Can you work these out from the model? Positions are in its coordinate system, mm. Face numbers are marked on the shaded views. Give positions to 0.01 mm unless a question says otherwise; leave off trailing zeros. Write each loop counter-clockwise with the first axis right and the second up, starting at its lowest first coordinate (ties: lowest second). Pieces come first, ordered by that corner, then holes. Notation, with made-up numbers: (55.25, 33.5) -> (86.25, 33.5) arc R24 cw to (86.25, 53.5) -> close; hole circle Ø9 at (12.5, 21.5). An arc over 180 degrees is marked (long way). One line per item, written item: value.
from build123d import *

# Parameters (mm, degrees)
F0_R     = 63.5
F1_DEPTH = 127


with BuildPart() as f1:
    # F0 (on Right) → F1 (new body)
    with BuildSketch(Plane.YZ):
        with BuildLine():
            Line((423.9281, 127), (-1100.0719, 127))
            ThreePointArc((-1100.0719, 127), (-1227.0719, 0), (-1100.0719, -127))
            Line((-1100.0719, -127), (423.9281, -127))
            ThreePointArc((423.9281, -127), (550.9281, 0), (423.9281, 127))
        make_face()
        with Locations((-1100.0719, 0)):
            Circle(F0_R, mode=Mode.SUBTRACT)
        with Locations((423.9281, 0)):
            Circle(F0_R, mode=Mode.SUBTRACT)
    extrude(amount=F1_DEPTH)


solid = f1.part
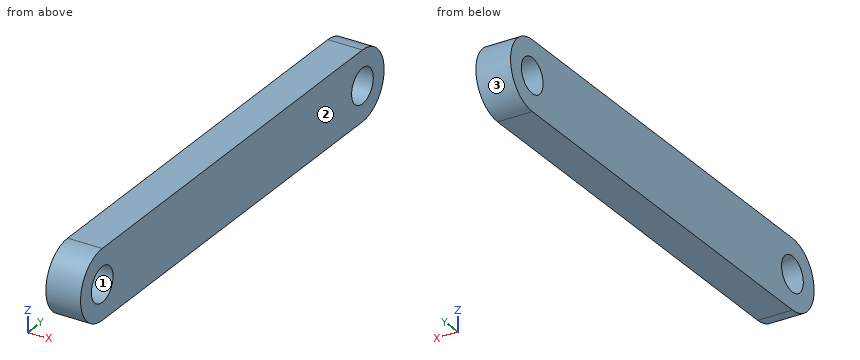
1) Will these pins go through, and if not, where does the flat tip stop? pin 1 (6 mm diameter, centred on x = 98, z = 62.5, fed in from -Y); pin 2 (10 mm diameter, centred on y = -617.5, z = -59, fed in from -X); pin 3 (2 mm diameter, centred on x = 57.5, z = -15.5, fed in from -Y); pin 4 (10 mm diameter, centred on x = 108.5, z = -38.5, fed in from +Y).
Answer list:
pin 1: stops at y = -1212.27
pin 2: stops at x = 0
pin 3: stops at y = -1226.24
pin 4: stops at y = 546.43
2) I need wall thicknesses on L1, parallel to Y at x = 63.5, z = -39.5; L2, parallel to Y at x = 92, z = 47; L3, parallel to Y at x = 112, z = 102. Which ranges of each line are inside material? Lowest first, please.
Answer list:
L1: y = -1220.77 to -1149.79, -1050.35 to 374.21, 473.65 to 544.63
L2: y = -1218.05 to -1142.77, -1057.37 to 381.23, 466.63 to 541.91
L3: y = -1175.74 to 499.59
3) If we section it at D-D (z = 111.5): Write out the boundary of the cut face in (x, y), and give its area (3 significant figures).
Answer list:
outline: (0, -1160.87) -> (127, -1160.87) -> (127, 484.73) -> (0, 484.73) -> close
area: 209,000 mm^2
4) If we section it at A-A (z = 0): Write out the boundary of the cut face in (x, y), and give its area (3 significant figures).
Answer list:
outline: (0, -1227.07) -> (127, -1227.07) -> (127, -1163.57) -> (0, -1163.57) -> close; (0, -1036.57) -> (127, -1036.57) -> (127, 360.43) -> (0, 360.43) -> close; (0, 487.43) -> (127, 487.43) -> (127, 550.93) -> (0, 550.93) -> close
area: 194,000 mm^2
5) If we section it at B-B (x = 103): Write out the boundary of the cut face in (y, z), and give its area (3 significant figures).
Answer list:
outline: (-1100.07, -127) -> (423.93, -127) arc R127 ccw to (423.93, 127) -> (-1100.07, 127) arc R127 ccw to start; hole circle Ø127 at (-1100.07, 0); hole circle Ø127 at (423.93, 0)
area: 412,000 mm^2
6) We'd pull the mould along Y, two halves only. Please class the marked faces 1, 2 and 3: released by +Y, released by -Y, zero draft, split by the parting line, or undercut.
Answer list:
face 1: undercut
face 2: zero draft
face 3: released by +Y
7) If we section it at C-C (z = -88): Write out the boundary of the cut face in (x, y), and give its area (3 significant figures).
Answer list:
outline: (0, -1191.64) -> (127, -1191.64) -> (127, 515.5) -> (0, 515.5) -> close
area: 217,000 mm^2
